Autodesk Inventor part; units mm, degrees
ref_plane "YZ Plane" through (0, 0, 0) normal (1, 0, 0) x (0, 1, 0)
ref_plane "XZ Plane" through (0, 0, 0) normal (0, 1, 0) x (-1, 0, 0)
ref_plane "XY Plane" through (0, 0, 0) normal (0, 0, 1) x (1, 0, 0)
sketch "Sketch3" plane through (0, 0, 0) normal (0, 1, 0) x (-1, 0, 0)
  line L0 (-25, 25) -> (25, 25)
  line L1 (25, 25) -> (25, -25)
  line L2 (25, -25) -> (-25, -25)
  line L3 (-25, -25) -> (-25, 25)
  line L4 (-25, 25) -> (25, -25) construction
  line L5 (25, 25) -> (-25, -25) construction
  point P0 (0, 0)
  dimension "d6" = 50
  dimension "d7" = 50
extrude "Extrusion2" add sketch "Sketch3" along normal blind 70
sketch "Sketch4" plane through (-25, 0, 25) normal (0, 0, 1) x (1, 0, 0)
  line L0 (50, 0) -> (0, 0)
  line L1 (0, 0) -> (25, 70)
  line L2 (50, 70) -> (0, 70)
  line L3 (0, 0) -> (0, 70)
  line L4 (0, 70) -> (0, 0)
  point P0 (25, 0)
extrude "Extrusion3" cut sketch "Sketch4" along normal through all both and the other way through all
mirror "Mirror1" about plane through (0, 0, 0) normal (1, 0, 0) of "Extrusion3"
sketch "Sketch5" plane through (0, 0, 0) normal (1, 0, 0) x (0, 1, 0)
  line L0 (70, -25) -> (70, 25)
  line L1 (70, 0) -> (70, -25)
  line L2 (70, -25) -> (0, -25)
  line L3 (0, -25) -> (70, 0)
  point P0 (0, 0)
extrude "Extrusion4" cut sketch "Sketch5" along normal through all both and the other way through all
mirror "Mirror2" about plane through (0, 0, 0) normal (0, 0, 1) of "Extrusion4"
properties part number "exp1"
For this review, take the finished solid that the model builds, in its own axes (mm). Round coordinates to 2 decimals unless told otherwise and drop trailing zeros. Write each loop counter-clockwise with the first axis right and the second up, starting at its lowest first coordinate (ties: lowest second). Pieces come first, ordered by that corner, then holes. Notation, with made-up numbers: (87.5, -34.75) -> (111.5, -34.75) arc R19 ccw to (111.5, -24.75) -> close; hole circle Ø7 at (36, -33). An arc over 180 degrees is marked (long way). Use CSV: the item, a comma, the result in double quotes.
(1) Consider section B-B, the plane x = -3.5. Give the boundary of the cut face in (y, z), plus the area to 3 significant figures.
Computed values:
outline,"(0, -25) -> (60.2, -3.5) -> (60.2, 3.5) -> (0, 25) -> close"
area,"1,720 mm²"
(2) Consider section A-A, the plane z = 4.5. Give the boundary of the cut face in (x, y).
Computed values:
outline,"(-25, 0) -> (25, 0) -> (4.5, 57.4) -> (-4.5, 57.4) -> close"
(3) Clearance check with flat-ended pins moving along their axes: P1, Ø1.5, axis at y = 26.5, z = 14.5, coming from the +X side; P2, Ø10, axis at x = 1.5, y = 53.5, coming from the +Z side; P3, Ø1, axis at y = 35.5, z = 3.5, coming from the +X side. State where each tip first meets the part, or that it passes through.
Computed values:
P1,"x = 15.8"
P2,"z = 7.68"
P3,"x = 12.5"
(4) To check wall thickness, follow L1, parallel to Z at x = -6.5, y = 47; L2, parallel to X at y = 28, z = -10; L3, parallel to Z at x = -16, y = 18. State the ranges of each line that lie inside material, in increasing order. Write a range as [from, to].
Computed values:
L1,"[-8.21, 8.21]"
L2,"[-15, 15]"
L3,"[-18.57, 18.57]"
